Source: CAD feature listing. Evaluate the final solid. Frame: model axes, mm. A direction names the side the tool comes from. Give positions to 0.01 mm unless a question says otherwise; leave off trailing zeros. Loops run counter-clockwise (first coordinate to the right, second up) from the corner with the lowest first, then second, coordinate; pieces in that order, holes last. Notation, with made-up numbers: (-27.5, 55) - (26.5, 55) arc R23 cw to (26.5, 84) - close; hole circle Ø10 at (-32, -11.75). An arc over 180 degrees is marked (long way). Put each result on its own line as item: value.
```python
from build123d import *

# Parameters (mm, degrees)
SKETCH005_W   = 54
SKETCH005_H   = 45
SKETCH005_R   = 3.5
SKETCH005_R_2 = 2.5
PAD001_DEPTH  = 5
FILLET_R      = 5
POCKET_DEPTH  = 5
SKETCH007_R   = 1.5
PAD002_DEPTH  = 4
CHAMFER_SIZE  = 3.99
FILLET001_R   = 12


with BuildPart() as part:
    # Sketch005 → Pad001 (new body)
    with BuildSketch(Plane.XZ):
        with Locations((0, 25.5)):
            Rectangle(SKETCH005_W, SKETCH005_H)
        with Locations((-20.3, 41)):
            Circle(SKETCH005_R, mode=Mode.SUBTRACT)
        with Locations((-20.3, 10)):
            Circle(SKETCH005_R, mode=Mode.SUBTRACT)
        with Locations((20.3, 10)):
            Circle(SKETCH005_R_2, mode=Mode.SUBTRACT)
        with Locations((20.3, 41)):
            Circle(SKETCH005_R_2, mode=Mode.SUBTRACT)
    extrude(amount=PAD001_DEPTH)

    # Fillet
    fillet_edges = [part.edges().sort_by_distance(p)[0] for p in [
        (-27, -2.5, 48),
        (-27, -2.5, 3),
        (27, -2.5, 48),
        (27, -2.5, 3),
    ]]
    fillet(fillet_edges, radius=FILLET_R)

    # Sketch006 (on Face2 of Fillet) → Pocket (cut)
    with BuildSketch(Plane(origin=(0, 0, 0), x_dir=(1, 0, 0), z_dir=(0, 1, 0))):
        Polygon((-7.315321, -17.05), (-7.315321, -13.95), (-10, -12.4), (-12.684679, -13.95), (-12.684679, -17.05), (-10, -18.6), align=None)
        Polygon((-7.315321, -33.95), (-10, -32.4), (-12.684679, -33.95), (-12.684679, -37.05), (-10, -38.6), (-7.315321, -37.05), align=None)
        Polygon((12.684679, -37.05), (12.684679, -33.95), (10, -32.4), (7.315321, -33.95), (7.315321, -37.05), (10, -38.6), align=None)
        Polygon((12.684679, -17.05), (12.684679, -13.95), (10, -12.4), (7.315321, -13.95), (7.315321, -17.05), (10, -18.6), align=None)
    extrude(amount=-POCKET_DEPTH, mode=Mode.SUBTRACT)

    # Sketch007 (on Face2 of Pocket) → Pad002 (join)
    with BuildSketch(Plane(origin=(0, 0, 0), x_dir=(1, 0, 0), z_dir=(0, 1, 0))):
        Polygon((-14, -3), (14, -3), (14, -24.5), (27, -24.5), (27, -28.5), (14, -28.5), (14, -48), (-14, -48), (-14, -27.5), (-27, -27.5), (-27, -23.5), (-14, -23.5), align=None)
        with Locations((-10, -15.5)):
            Circle(SKETCH007_R, mode=Mode.SUBTRACT)
        with Locations((10, -15.5)):
            Circle(SKETCH007_R, mode=Mode.SUBTRACT)
        with Locations((-10, -35.5)):
            Circle(SKETCH007_R, mode=Mode.SUBTRACT)
        with Locations((10, -35.5)):
            Circle(SKETCH007_R, mode=Mode.SUBTRACT)
    extrude(amount=PAD002_DEPTH)

    # Chamfer
    chamfer_edges = [part.edges().sort_by_distance(p)[0] for p in [
        (27, 4, 26.5),
        (-27, 4, 25.5),
    ]]
    chamfer(chamfer_edges, length=CHAMFER_SIZE)

    # Fillet001
    fillet001_edges = [part.edges().sort_by_distance(p)[0] for p in [
        (23.01, 4, 26.5),
        (-23.01, 4, 25.5),
    ]]
    fillet(fillet001_edges, radius=FILLET001_R)


with BuildPart() as part_1:
    # Body005 placement: moved
    add(part.part.moved(Location((0, 16.5, 0))))


solid = part_1.part
```
1) Access query for faces 4 (the flat face through (-8.68, 14.04, 37.84)), 5 (the flat face through (-19, 18, 27.5)), 6 (the flat face through (19, 18, 28.5)). Directions: +Z, -Z, +X, -X, +Y, -Y. A direction counts if a zero-diameter tool reaches every point of the face in a straight line with its end or side. Return the directions, or none.
Check result:
face 4: -Y
face 5: +Z, -X, +Y
face 6: +Z, +X, +Y
2) Mould query, pull axis X, two halves, no side actions, for faces 1 (the flat face through (27, 14, 25)), 2 (the flat face through (-11.361, 14.035, 37.814)), 3 (the flat face through (0, 15, 3)). Classes: pulls with the +X half, pulls with the -X half, needs draft (parallel to the pull), parting line crosses it, or undercut.
Check result:
face 1: pulls with the +X half
face 2: undercut
face 3: needs draft
3) Section query C-C, the plane y = 19.5. Output: boundary loops of the cut face in (x, z), plus the area to 3 significant figures.
Check result:
outline: (-22.84, 23.5) - (-14, 23.5) - (-14, 3) - (14, 3) - (14, 24.5) - (22.84, 24.5) - (22.84, 28.5) - (14, 28.5) - (14, 48) - (-14, 48) - (-14, 27.5) - (-22.84, 27.5) - close; hole circle Ø3 at (-10, 15.5); hole circle Ø3 at (-10, 35.5); hole circle Ø3 at (10, 15.5); hole circle Ø3 at (10, 35.5)
area: 1,300 mm²
4) Section query B-B, the plane x = -20.3. Output: boundary loops of the cut face in (y, z), plus the area to 3 significant figures.
Check result:
outline: (11.5, 3) - (16.5, 3) - (16.5, 6.5) - (11.5, 6.5) - close; (11.5, 13.5) - (16.5, 13.5) - (16.5, 23.5) - (20.29, 23.5) - (20.29, 27.5) - (16.5, 27.5) - (16.5, 37.5) - (11.5, 37.5) - close; (11.5, 44.5) - (16.5, 44.5) - (16.5, 48) - (11.5, 48) - close
area: 170 mm²
5) Section query A-A, the plane z = 41. Output: boundary loops of the cut face in (x, y), plus the area to 3 significant figures.
Check result:
outline: (-27, 11.5) - (-23.8, 11.5) - (-23.8, 16.5) - (-27, 16.5) - close; (-16.8, 11.5) - (17.8, 11.5) - (17.8, 16.5) - (14, 16.5) - (14, 20.5) - (-14, 20.5) - (-14, 16.5) - (-16.8, 16.5) - close; (22.8, 11.5) - (27, 11.5) - (27, 16.5) - (22.8, 16.5) - close
area: 322 mm²
6) Section query D-D, the plane z = 25.5. Output: boundary loops of the cut face in (x, y).
Check result:
outline: (-27, 11.5) - (27, 11.5) - (27, 16.51) - (26.52, 16.99) arc R12 ccw to (18.04, 20.5) - (-18.04, 20.5) arc R12 ccw to (-26.52, 16.99) - (-27, 16.51) - close
7) Pin query (flat end, axial travel): P1, Ø4, axis at y = 19, z = 15.5, coming from the -X side; P2, Ø4, axis at x = 22, z = 40.5, coming from the +Y side; P3, Ø1.2, axis at x = 19.5, y = 18, coming from the -Z side; P4, Ø1.8, axis at x = 10, z = 35.5, coming from the +Y side. Return the tip coordinate at first contact, or that it passes through.
Check result:
P1: x = -14
P2: y = 16.5
P3: z = 24.5
P4: through
8) Material intervals for line 1 along Z through (x, y) = (-20.3, 14.8); line 2 along Z through (x, y) = (-10, 18.4); line 3 along X through (y, z) = (17.95, 35.5), sorted ascending. Write a range as [from, to].
Check result:
line 1: [3, 6.5], [13.5, 37.5], [44.5, 48]
line 2: [3, 14], [17, 34], [37, 48]
line 3: [-14, -11.5], [-8.5, 8.5], [11.5, 14]
